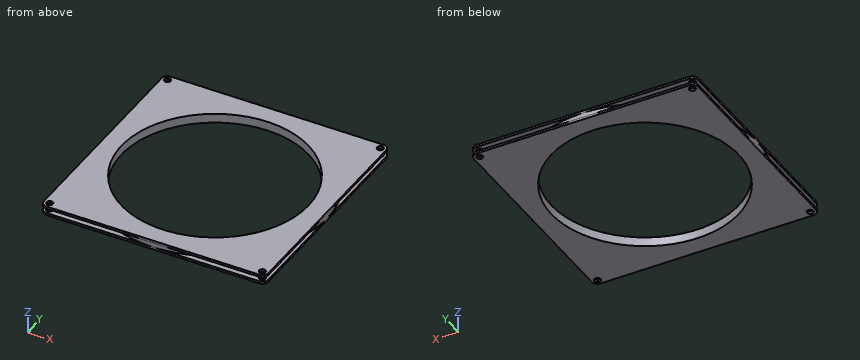
```python
from build123d import *

# Parameters (mm, degrees)
F0_W     = 152.4
F0_H     = 152.4
F0_R     = 2.15265
F0_R_2   = 63.5
F1_DEPTH = 1.5875
F2_R     = 76.2
F2_R_2   = 63.5
F3_DEPTH = 3.175
F4_W     = 152.4
F4_H     = 152.4
F4_R     = 2.15265
F4_R_2   = 63.5
F5_DEPTH = 1.5875
F6_R     = 3.96875


with BuildPart() as f1:
    # F0 (on Top) → F1 (new body)
    with BuildSketch(Plane.XY):
        Rectangle(F0_W, F0_H)
        with Locations((-72.23125, -72.23125)):
            Circle(F0_R, mode=Mode.SUBTRACT)
        with Locations((72.23125, -72.23125)):
            Circle(F0_R, mode=Mode.SUBTRACT)
        with Locations((-72.23125, 72.23125)):
            Circle(F0_R, mode=Mode.SUBTRACT)
        Circle(F0_R_2, mode=Mode.SUBTRACT)
        with Locations((72.23125, 72.23125)):
            Circle(F0_R, mode=Mode.SUBTRACT)
    extrude(amount=F1_DEPTH)

    # F2 (on face) → F3 (join)
    with BuildSketch(Plane.XY.offset(1.5875)):
        Circle(F2_R)
        Circle(F2_R_2, mode=Mode.SUBTRACT)
    extrude(amount=F3_DEPTH)

    # F4 (on face) → F5 (join)
    with BuildSketch(Plane.XY.offset(4.7625)):
        Rectangle(F4_W, F4_H)
        with Locations((-72.23125, -72.23125)):
            Circle(F4_R, mode=Mode.SUBTRACT)
        with Locations((72.23125, -72.23125)):
            Circle(F4_R, mode=Mode.SUBTRACT)
        with Locations((-72.23125, 72.23125)):
            Circle(F4_R, mode=Mode.SUBTRACT)
        Circle(F4_R_2, mode=Mode.SUBTRACT)
        with Locations((72.23125, 72.23125)):
            Circle(F4_R, mode=Mode.SUBTRACT)
    extrude(amount=F5_DEPTH)

    # F6
    f6_edges = [f1.edges().sort_by_distance(p)[0] for p in [
        (-76.2, 76.2, 0.79375),
        (-76.2, -76.2, 0.79375),
        (76.2, -76.2, 0.79375),
        (76.2, 76.2, 0.79375),
        (-76.2, 76.2, 5.55625),
        (-76.2, -76.2, 5.55625),
        (76.2, -76.2, 5.55625),
        (76.2, 76.2, 5.55625),
    ]]
    fillet(f6_edges, radius=F6_R)


solid = f1.part
```
CAD build for the part. Positions are in the model's coordinates, mm. Coordinates: 2 decimals unless noted, no trailing zeros. Write each loop counter-clockwise with the first axis right and the second up, starting at its lowest first coordinate (ties: lowest second). Pieces come first, ordered by that corner, then holes.
(1) Cut at A-A, the plane x = 7.5. List the corners of the cut face in (y, z).
(2) Flat gauge pin, fed straight in: pin 1 (2.5 mm diameter, centred on x = -72.23, y = 72.23, fed in from -Z). Where does the tip first touch, or does it go through?
(3) Cut at B-B, the plane y = 23. List the corners of the cut face in (x, z).
(4) Drill centre lines: probe 1 along Z at (x, y) = (53, 56); probe 2 along Y at (x, z) = (-0.5, 1.5); probe 3 along X at (y, z) = (24.5, 3.25). Where is each one in solid material? Low to high.
Geometry says:
1. outline: (-76.2, 0) - (-63.06, 0) - (-63.06, 6.35) - (-76.2, 6.35) - (-76.2, 4.76) - (-75.83, 4.76) - (-75.83, 1.59) - (-76.2, 1.59) - close; (63.06, 0) - (76.2, 0) - (76.2, 1.59) - (75.83, 1.59) - (75.83, 4.76) - (76.2, 4.76) - (76.2, 6.35) - (63.06, 6.35) - close
2. pin 1: passes through
3. outline: (-76.2, 0) - (-59.19, 0) - (-59.19, 6.35) - (-76.2, 6.35) - (-76.2, 4.76) - (-72.65, 4.76) - (-72.65, 1.59) - (-76.2, 1.59) - close; (59.19, 0) - (76.2, 0) - (76.2, 1.59) - (72.65, 1.59) - (72.65, 4.76) - (76.2, 4.76) - (76.2, 6.35) - (59.19, 6.35) - close
4. probe 1: z = 0 to 1.59, 4.76 to 6.35
4. probe 2: y = -76.2 to -63.5, 63.5 to 76.2
4. probe 3: x = -72.15 to -58.58, 58.58 to 72.15
